Autodesk Inventor part; units mm, degrees
ref_plane "Work Plane1" through (0, 30, -41.5) normal (0, 0, 1) x (1, 0, 0)
ref_plane "YZ Plane" through (0, 0, 0) normal (1, 0, 0) x (0, 1, 0)
ref_plane "XZ Plane" through (0, 0, 0) normal (0, 1, 0) x (-1, 0, 0)
sketch "Sketch1" plane through (0, 0, 0) normal (0, 0, 1) x (1, 0, 0)
  arc A0 (-35.9893, 3.2169) -> (-30.1047, 1.1907) centre (-32.6581, 3.3332) ccw
  line L0 (-30.1047, 1.1907) -> (-16, 18)
  line L1 (-41.5, 35) -> (-41.5, 25)
  line L2 (-41.5, 25) -> (-36.75, 25)
  line L3 (0, 0) -> (0, 35) construction
  line L4 (0, 0) -> (-46.1303, 0) construction
  line L5 (-16, 18) -> (-16, 35)
  line L6 (-16, 35) -> (-41.5, 35)
  line L7 (-16, 18) -> (0, 18)
  line L8 (0, 18) -> (0, 35)
  line L9 (-16, 35) -> (0, 35)
  line L10 (-41.5, 35) -> (-41.1508, 45)
  line L11 (-41.1508, 45) -> (-31.1508, 45)
  line L12 (-31.1508, 45) -> (-30.2759, 35)
  line L13 (-36.75, 25) -> (-35.9893, 3.2169)
  dimension "d0" = 32
  dimension "d2" = 18
  dimension "d4" = 83
  dimension "d20" = 35
  dimension "d21" = 140
  dimension "d22" = 10
  dimension "d44" = 95
  dimension "d45" = 10
  dimension "d46" = 92
  dimension "d48" = 73.5
  dimension "d49" = 92
  dimension "d73" = 45
revolve "Revolution1" add sketch "Sketch1" angle 360 about axis through (0, 0, 0) along (0, 1, 0)
fillet "Fillet1" radius 10 1 edges at (30.2759, 35, 0)
sketch "Sketch3" plane through (0, 18, 0) normal (0, -1, 0) x (1, 0, 0)
  circle A0 centre (-6, 0) radius 1.6
  circle A1 centre (6, 0) radius 1.6
  circle A2 centre (0, 13) radius 1.6
  circle A3 centre (-11.2583, 6.5) radius 1.6
  circle A4 centre (-11.2583, -6.5) radius 1.6
  circle A5 centre (0, -13) radius 1.6
  circle A6 centre (11.2583, -6.5) radius 1.6
  circle A7 centre (11.2583, 6.5) radius 1.6
  point P0 (0, 0)
  dimension "d50" = 3.2
  dimension "d51" = 3.2
  dimension "d52" = 6
  dimension "d53" = 6
  dimension "d54" = 3.2
  dimension "d55" = 13
  dimension "d58" = 360
extrude "Extrusion1" cut sketch "Sketch3" against normal through all contours A0 | A1 | A2 | A5
sketch "Sketch4" plane through (0, 18, 0) normal (0, -1, 0) x (1, 0, 0)
  circle A0 centre (0, 0) radius 10
  circle A1 centre (-6, 0) radius 1.6
  circle A2 centre (6, 0) radius 1.6
  point P0 (0, 0)
  dimension "d62" = 20
extrude "Extrusion2" add sketch "Sketch4" along normal blind 5
ref_plane "Work Plane1" through (0, 30, -41.5) normal (0, 0, 1) x (1, 0, 0)
equation "\"d51\" = d50"
properties part number "020" material "Concrete"
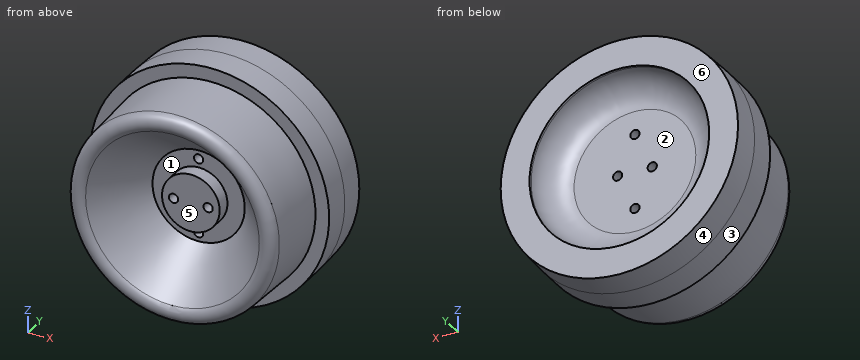
The listing builds one solid part. Answer for the finished solid, in the listing's coordinates (mm). Face numbers are marked on the shaded views. A direction names the side the tool comes from. Round coordinates to 2 decimals unless told otherwise and drop trailing zeros. Loops run counter-clockwise (first coordinate to the right, second up) from the corner with the lowest first, then second, coordinate; pieces in that order, holes last.
Q1. Find the intervals of material crossed by line 1 (Z direction, x = 0, y = 26); line 2 (X direction, y = 14, z = -16.5); line 3 (Y direction, x = -24.5, z = 28), in increasing order.
Q2. Section D-D, the plane y = 11 is taken. Determine the outline of the cut face in (x, z).
Q3. Section C-C, the plane y = 29 is taken. Determine the outline of the cut face in (x, z).
Q4. For a pull along Z with two mould halves and no side action, classify the marked faces 4, 5 and 6 as released by +Z, released by -Z, zero draft, split by the parting line, or undercut.
Q5. Which of the six approach directions +Z, -Z, +X, -X, +Y, -Y give full straight-line access (tool end or side, diameter ignored) to the marked faces 1, 2 and 3?
Q6. Section A-A, the plane x = 0 is taken. Count the separate pieces of the cut face and the enclosed holes in it, then the cut area to 3 significant figures.
Q7. Given pin 1 Ø5 at (x, z) = (0, -13) entering from +Y; pin 2 Ø4 at (x, z) = (-6, 0) entering from -Y; pin 3 Ø3 at (x, z) = (24, -14) entering from +Y, each flat-ended and moving along its own axis, determine where each tip first touches the part or whether it passes through.
Completed:
1. line 1: z = -41.5 to -14.6, -11.4 to 11.4, 14.6 to 41.5
1. line 2: x = -32.41 to -10.12, 10.12 to 32.41
1. line 3: y = 25 to 45
2. outline: circle Ø72.52 at (0, 0); hole circle Ø43.75 at (0, 0)
3. outline: circle Ø83 at (0, 0); hole circle Ø3.2 at (-6, 0); hole circle Ø3.2 at (0, -13); hole circle Ø3.2 at (0, 13); hole circle Ø3.2 at (6, 0)
4. face 4: split by the parting line
4. face 5: undercut
4. face 6: zero draft
5. face 1: -Y
5. face 2: +Y
5. face 3: +Y, -Y
6. separate pieces: 3
6. enclosed holes: 0
6. area: 2,030 mm2
7. pin 1: stops at y = 35
7. pin 2: stops at y = 13
7. pin 3: stops at y = 39.24
